Read the model definition and answer for the solid it produces. Units are mm, in the model's axes. Face numbers are marked on the shaded views. A direction names the side the tool comes from. Coordinates: 2 decimals unless noted, no trailing zeros. Order: outer loops, then holes, each group sorted by start corner. A loop starts at its lowest first (then second) coordinate and runs counter-clockwise, first axis right, second up. Notation, with made-up numbers: (2.25, -9) -> (32.25, -9) arc R36 cw to (32.25, 29) -> close; hole circle Ø8 at (76.25, 69). An arc over 180 degrees is marked (long way). Use CSV: the item, a comma, the result in double quotes.
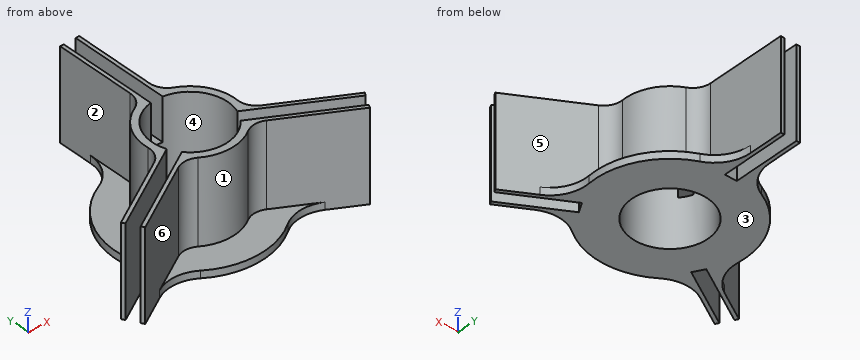
```python
from build123d import *

# Parameters (mm, degrees)
SKETCH1_R                       = 20.75
BOSS_EXTRUDE1_DEPTH             = 50
BOSS_EXTRUDE2_DEPTH             = 3.2
THICKEN1_OUTLINE_R              = 24.85
THICKEN1_OUTLINE_R_2            = 20.85
THICKEN1_DEPTH                  = 50
THICKEN2_OUTLINE_W              = 2
THICKEN2_OUTLINE_H              = 37
THICKEN2_DEPTH                  = 50
THICKEN2_START                  = 26.35
THICKEN2_2_DEPTH                = 23.65
THICKEN3_OUTLINE_W              = 2
THICKEN3_OUTLINE_H              = 37
THICKEN3_DEPTH                  = 50
THICKEN3_START                  = 26.35
THICKEN3_2_DEPTH                = 23.65
BOSS_EXTRUDE4_REACH             = 95.501
SKETCH4_W                       = 26.35
SKETCH4_H                       = 17.15
BOSS_EXTRUDE4_DIRECTION_2_REACH = 95.501
FILLET1_R                       = 10
SKETCH3_R                       = 41.5
BOSS_EXTRUDE3_DEPTH             = 4
FILLET2_R                       = 20
CIRPATTERN4_COUNT               = 3
MOVE_FACE3_BY                   = 0.25
MOVE_FACE4_BY                   = 0.1
MOVE_FACE4_2_BY                 = 0.1
MOVE_FACE4_3_BY                 = 0.1
MOVE_START                      = 26.35
MOVE_FACE5_OUTLINE_W            = 6.6
MOVE_FACE5_OUTLINE_H            = 20.75
MOVE_FACE5_DEPTH                = 23.65
CIRPATTERN1_COUNT               = 3


with BuildPart() as part:
    # Sketch1 → Boss-Extrude1 (new body)
    with BuildSketch(Plane.XY):
        Circle(SKETCH1_R)
    extrude(amount=BOSS_EXTRUDE1_DEPTH)

    # Move Face3: a curved face moved outward by 0.25
    add(Solid.thicken(part.faces().sort_by_distance((-20.75, 0, 25))[0], MOVE_FACE3_BY))


with BuildPart() as body_2:
    # Sketch2 → Boss-Extrude2 (new, symmetric)
    with BuildSketch(Plane(origin=(0, 0, 0), x_dir=(0, 0, -1), z_dir=(1, 0, 0))):
        Polygon((-26.35, 20.75), (-26.35, 38), (0, 38), (0, 75), (-50, 75), (-50, 20.75), align=None)
    extrude(amount=BOSS_EXTRUDE2_DEPTH, both=True)

    # Move Face4: a face moved outward by 0.1
    extrude(body_2.faces().sort_by_distance((0, 38, 13.175))[0], amount=MOVE_FACE4_BY, dir=(0, -1, 0))

    # Move Face4 2: a face moved outward by 0.1
    extrude(body_2.faces().sort_by_distance((-3.2, 51.599129054, 27.380423031))[0], amount=MOVE_FACE4_2_BY, dir=(-1, 0, 0))

    # Move Face4 3: a face moved outward by 0.1
    extrude(body_2.faces().sort_by_distance((3.2, 51.599129054, 27.380423031))[0], amount=MOVE_FACE4_3_BY, dir=(1, 0, 0))

    # Move Face5: read off the stored shape, not the designer's step
    # Move Face5 outline → Move Face5 (add)
    with BuildSketch(Plane.XY.offset(MOVE_START)):
        with Locations((0, 10.375)):
            Rectangle(MOVE_FACE5_OUTLINE_W, MOVE_FACE5_OUTLINE_H)
    extrude(amount=MOVE_FACE5_DEPTH)


with BuildPart() as body_3:
    # Thicken1: read off the stored shape, not the designer's step
    # Thicken1 outline → Thicken1 (new body)
    with BuildSketch(Plane.XY):
        Circle(THICKEN1_OUTLINE_R)
        Circle(THICKEN1_OUTLINE_R_2, mode=Mode.SUBTRACT)
    extrude(amount=THICKEN1_DEPTH)

    # Thicken2: read off the stored shape, not the designer's step
    # Thicken2 outline → Thicken2 (add)
    with BuildSketch(Plane.XY):
        with Locations((-4.3, 56.5)):
            Rectangle(THICKEN2_OUTLINE_W, THICKEN2_OUTLINE_H)
    extrude(amount=THICKEN2_DEPTH)

    # Thicken2 2 outline → Thicken2 2 (add)
    with BuildSketch(Plane.XY.offset(THICKEN2_START)):
        with BuildLine():
            Line((-5.3, 38), (-5.3, 24.27823099))
            ThreePointArc((-5.3, 24.27823099), (-4.303593806, 24.474508787), (-3.3, 24.629910678))
            Line((-3.3, 24.629910678), (-3.3, 38))
            Line((-3.3, 38), (-5.3, 38))
        make_face()
    extrude(amount=THICKEN2_2_DEPTH)

    # Thicken3: read off the stored shape, not the designer's step
    # Thicken3 outline → Thicken3 (add)
    with BuildSketch(Plane.XY):
        with Locations((4.3, 56.5)):
            Rectangle(THICKEN3_OUTLINE_W, THICKEN3_OUTLINE_H)
    extrude(amount=THICKEN3_DEPTH)

    # Thicken3 2 outline → Thicken3 2 (add)
    with BuildSketch(Plane.XY.offset(THICKEN3_START)):
        with BuildLine():
            Line((5.3, 38), (3.3, 38))
            Line((3.3, 38), (3.3, 24.629910678))
            ThreePointArc((3.3, 24.629910678), (4.303593806, 24.474508787), (5.3, 24.27823099))
            Line((5.3, 24.27823099), (5.3, 38))
        make_face()
    extrude(amount=THICKEN3_2_DEPTH)

    # Boss-Extrude4: up to this face of the body (flat: up to its plane)
    boss_extrude4_end = Plane(body_3.part.faces().sort_by_distance((5.3, 52.715205781, 26.966203656))[0])
    # Sketch4 → Boss-Extrude4 (add, up to the picked face)
    with BuildSketch(Plane(origin=(0, 0, 0), x_dir=(0, 0, -1), z_dir=(1, 0, 0)), mode=Mode.PRIVATE) as boss_extrude4_sk1:
        with Locations((-13.175, 29.425)):
            Rectangle(SKETCH4_W, SKETCH4_H)
    boss_extrude4_tool1 = split(extrude(boss_extrude4_sk1.sketch, amount=BOSS_EXTRUDE4_REACH, mode=Mode.PRIVATE), bisect_by=boss_extrude4_end, keep=Keep.BOTH, mode=Mode.PRIVATE)
    add(boss_extrude4_tool1.solids().sort_by(Axis((0, 29.425, 13.175), (1, 0, 0)))[0])

    # Boss-Extrude4 direction 2: up to this face of the body (flat: up to its plane)
    boss_extrude4_direction_2_end = Plane(body_3.part.faces().sort_by_distance((-5.3, 52.715205781, 26.966203656))[0])
    # Sketch4 → Boss-Extrude4 direction 2 (add, up to the picked face)
    with BuildSketch(Plane(origin=(0, 0, 0), x_dir=(0, 0, -1), z_dir=(1, 0, 0)), mode=Mode.PRIVATE) as boss_extrude4_direction_2_sk1:
        with Locations((-13.175, 29.425)):
            Rectangle(SKETCH4_W, SKETCH4_H)
    boss_extrude4_direction_2_tool1 = split(extrude(boss_extrude4_direction_2_sk1.sketch, amount=-BOSS_EXTRUDE4_DIRECTION_2_REACH, mode=Mode.PRIVATE), bisect_by=boss_extrude4_direction_2_end, keep=Keep.BOTH, mode=Mode.PRIVATE)
    add(boss_extrude4_direction_2_tool1.solids().sort_by(Axis((0, 29.425, 13.175), (-1, 0, 0)))[0])

    # Fillet1
    fillet1_edges = [body_3.edges().sort_by_distance(p)[0] for p in [
        (-5.3, 24.27823099, 13.175),
        (5.3, 24.27823099, 13.175),
    ]]
    fillet(fillet1_edges, radius=FILLET1_R)

    # Sketch3 → Boss-Extrude3 (add)
    with BuildSketch(Plane.XY):
        Circle(SKETCH3_R)
    extrude(amount=BOSS_EXTRUDE3_DEPTH)

    # Fillet2
    fillet2_edges = [body_3.edges().sort_by_distance(p)[0] for p in [
        (-5.3, 41.160174927, 2),
        (5.3, 41.160174927, 2),
    ]]
    fillet(fillet2_edges, radius=FILLET2_R)


with BuildPart() as cirpattern4_1:
    # CirPattern4: pattern copy
    add(body_3.part.rotate(Axis((0, 0, 0), (0, 0, 1)), 1 * 360 / CIRPATTERN4_COUNT))


with BuildPart() as cirpattern4_2:
    # CirPattern4: pattern copy
    add(body_3.part.rotate(Axis((0, 0, 0), (0, 0, 1)), 2 * 360 / CIRPATTERN4_COUNT))

    # Combine2: read off the stored shape, not the designer's step
    # Combine2: union CirPattern4_1, body 3
    add(cirpattern4_1.part)
    add(body_3.part)


with BuildPart() as cirpattern1_1:
    # CirPattern1: pattern copy
    add(body_2.part.rotate(Axis((0, 0, 0), (0, 0, 1)), 1 * 360 / CIRPATTERN1_COUNT))


with BuildPart() as cirpattern1_2:
    # CirPattern1: pattern copy
    add(body_2.part.rotate(Axis((0, 0, 0), (0, 0, 1)), 2 * 360 / CIRPATTERN1_COUNT))


with BuildPart() as cirpattern4_2_1:
    add(cirpattern4_2.part)

    # Combine3: read off the stored shape, not the designer's step
    # Combine3: cut CirPattern1_2, CirPattern1_1, body 2, part
    add(cirpattern1_2.part, mode=Mode.SUBTRACT)
    add(cirpattern1_1.part, mode=Mode.SUBTRACT)
    add(body_2.part, mode=Mode.SUBTRACT)
    add(part.part, mode=Mode.SUBTRACT)


solid = cirpattern4_2_1.part
```
Item 1: Find section D-D, the plane z = 32. Give the number of separate pieces and of enclosed holes in the cut face, then the cut area to 3 significant figures.
Return value:
separate pieces,"3"
enclosed holes,"0"
area,"1,130 mm^2"
Item 2: Find section B-B, the plane x = 0. Give the vertices of the cut face in (y, z), then the cut area to 3 significant figures.
Return value:
outline,"(-41.5, 0) -> (-21, 0) -> (-21, 50) -> (-24.85, 50) -> (-24.85, 4) -> (-41.5, 4) -> close; (21, 0) -> (37.9, 0) -> (37.9, 26.35) -> (21, 26.35) -> close"
area,"704 mm^2"
Item 3: Each of these flat-tipped pins is pushed along its axis until it touches: P1, Ø8, axis at y = 32.5, z = 16.5, coming from the -X side; P2, Ø4.5, axis at x = -24.5, y = -12, coming from the +Z side; P3, Ø10, axis at y = -21.5, z = 36, coming from the -X side; P4, Ø25, axis at y = 35.5, z = 34.5, coming from the +X side. Where does it stop, or does it pass through?
Return value:
P1,"stops at x = -5.7"
P2,"stops at z = 50"
P3,"stops at x = -56.5"
P4,"stops at x = 9.74"
Item 4: Straight lines are drawn through the part: line 1 along Y through (x, z) = (0, 22); line 2 along X through (y, z) = (0, 34); line 3 along X through (y, z) = (35, 47.5). For each, find the intervals that lie inside material, in ascending order.
Return value:
line 1,"y = -24.85 to -21, 21 to 37.9"
line 2,"x = -24.85 to -21, 21 to 24.85"
line 3,"x = -5.3 to -3.3, 3.3 to 5.3"
Item 5: A tool of negligible diameter and unlimited length cuts with its end or side. For the marked faces 1, 2 and 3, from which of +Z, -Z, +X, -X, +Y, -Y can it reach the whole face along a straight path? Write none if from no direction.
Return value:
face 1,"+Z, -Y"
face 2,"+Z, -X, +Y"
face 3,"-Z, +X, -X, +Y, -Y"
Item 6: Find section A-A, the plane y = 0. Give the vertices of the cut face in (x, z), then the cut area to 3 significant figures.
Return value:
outline,"(-41.5, 0) -> (-21, 0) -> (-21, 50) -> (-24.85, 50) -> (-24.85, 4) -> (-41.5, 4) -> close; (21, 0) -> (41.5, 0) -> (41.5, 4) -> (24.85, 4) -> (24.85, 50) -> (21, 50) -> close"
area,"518 mm^2"
Item 7: The mould has two halves that part along Y. Classify the marked faces 4, 5 and 6: +Y half, -Y half, draft (parallel to the pull), parting line (faces both ways), or undercut.
Return value:
face 4,"undercut"
face 5,"+Y half"
face 6,"-Y half"
